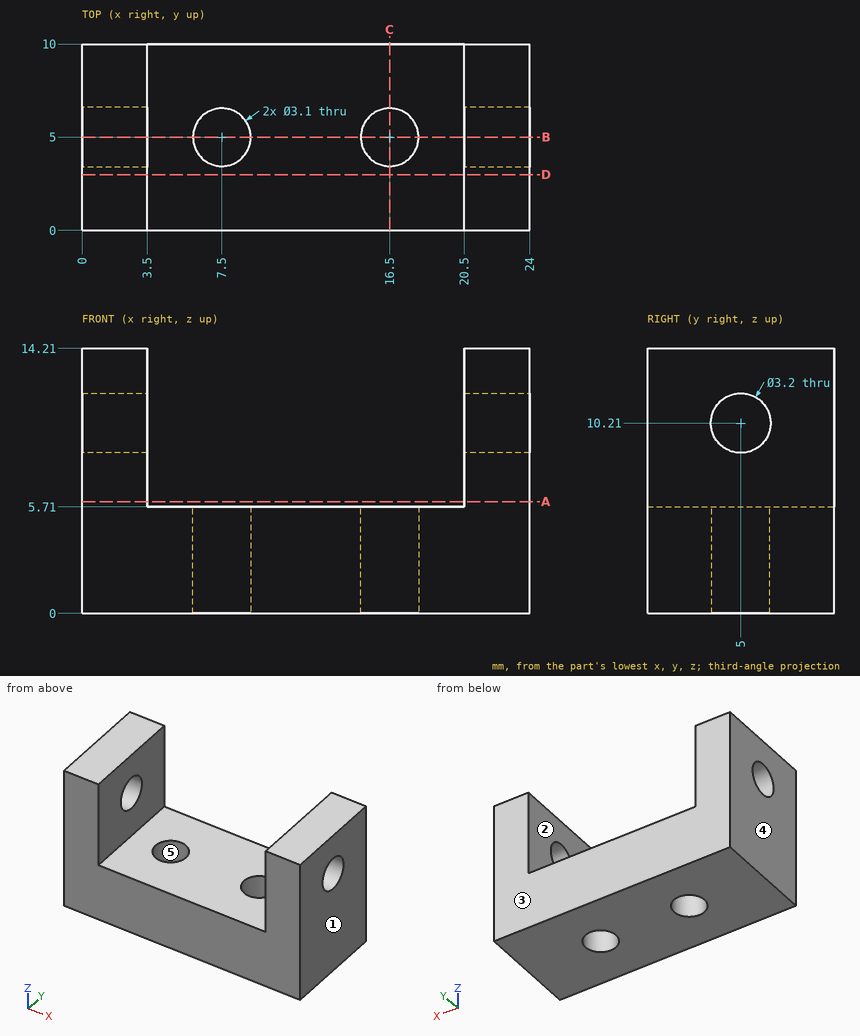
Can you work these out from the drawing? Everything is in mm from the part's minimum corner. A direction names the side the tool comes from. Coordinates: 2 decimals unless noted, no trailing zeros. Write each loop counter-clockwise with the first axis right and the second up, starting at its lowest first coordinate (ties: lowest second). Pieces come first, ordered by that corner, then holes. Notation, with made-up numbers: (-4.75, -34) - (43.25, -34) arc R10 cw to (43.25, -21) - close; hole circle Ø11 at (32.5, 33.25). An arc over 180 degrees is marked (long way). One line per item, written item: value.
1) Suppose I cut it at D-D on y = 3. Write out the boundary of the cut face in (x, z).
Model answer:
outline: (0, 0) - (24, 0) - (24, 14.21) - (20.5, 14.21) - (20.5, 5.71) - (3.5, 5.71) - (3.5, 14.21) - (0, 14.21) - close
2) We'd pull the mould along Y, two halves only. Please class the marked faces 3, 4 and 5: pulls with the +Y half, pulls with the -Y half, needs draft (parallel to the pull), parting line crosses it, or undercut.
Model answer:
face 3: pulls with the +Y half
face 4: needs draft
face 5: undercut
3) Suppose I cut it at A-A on z = 6. Write out the boundary of the cut face in (x, y).
Model answer:
outline: (0, 0) - (3.5, 0) - (3.5, 10) - (0, 10) - close; (20.5, 0) - (24, 0) - (24, 10) - (20.5, 10) - close
4) I'm going to push a flat-ended pin straight in: P1, Ø3, axis at x = 10.5, y = 4, coming from the +Z side. Where does the tip first touch, or does it pass through?
Model answer:
P1: stops at z = 5.71
5) Suppose I cut it at C-C on x = 16.5. Write out the boundary of the cut face in (y, z).
Model answer:
outline: (0, 0) - (3.45, 0) - (3.45, 5.71) - (0, 5.71) - close; (6.55, 0) - (10, 0) - (10, 5.71) - (6.55, 5.71) - close
6) I need wall thicknesses on line 1 along Y through (x, z) = (1.05, 10.21); line 2 along X through (y, z) = (5.5, 4); line 3 along X through (y, z) = (0.5, 12.75). Which ranges of each line are inside material? Lowest first, please.
Model answer:
line 1: y = 0 to 3.4, 6.6 to 10
line 2: x = 0 to 6.03, 8.97 to 15.03, 17.97 to 24
line 3: x = 0 to 3.5, 20.5 to 24
7) Suppose I cut it at B-B on y = 5. Write out the boundary of the cut face in (x, z).
Model answer:
outline: (0, 0) - (5.95, 0) - (5.95, 5.71) - (3.5, 5.71) - (3.5, 8.61) - (0, 8.61) - close; (0, 11.81) - (3.5, 11.81) - (3.5, 14.21) - (0, 14.21) - close; (9.05, 0) - (14.95, 0) - (14.95, 5.71) - (9.05, 5.71) - close; (18.05, 0) - (24, 0) - (24, 8.61) - (20.5, 8.61) - (20.5, 5.71) - (18.05, 5.71) - close; (20.5, 11.81) - (24, 11.81) - (24, 14.21) - (20.5, 14.21) - close
8) On a 3-axis mill with a long thin cutter (end or side, diameter ignored), from which of +Z, -Z, +X, -X, +Y, -Y can I reach the whole of each face in a straight line? I mean the marked faces 1 and 2. Say none if no direction works.
Model answer:
face 1: +Z, -Z, +X, +Y, -Y
face 2: +Z, +Y, -Y
